Work out the finished part from the listing and answer in its coordinate system (mm). A direction names the side the tool comes from. Coordinates: 2 decimals unless noted, no trailing zeros. Loops run counter-clockwise (first coordinate to the right, second up) from the corner with the lowest first, then second, coordinate; pieces in that order, holes last. Notation, with made-up numbers: (-4.75, 74.25) -> (19.25, 74.25) arc R19 cw to (19.25, 100.25) -> close; hole circle Ø10 at (5, -10). An arc over 180 degrees is marked (long way). One line per question, with ' | ' between items.
```python
from build123d import *

# Parameters (mm, degrees)
F0_R     = 10
F0_R_2   = 5
F1_DEPTH = 10
F3_DEPTH = 15
F4_W     = 10
F4_H     = 5
F5_DEPTH = 35.001


with BuildPart() as f1:
    # F0 (on Front) → F1 (new body, symmetric)
    with BuildSketch(Plane.XZ):
        Circle(F0_R)
        Circle(F0_R_2, mode=Mode.SUBTRACT)
    extrude(amount=F1_DEPTH, both=True)

    # F2 (on face) → F3 (join)
    with BuildSketch(Plane(origin=(0, 10, 0), x_dir=(-1, 0, 0), z_dir=(0, 1, 0))):
        with BuildLine():
            ThreePointArc((0, -10), (-10, 0), (0, 10))
            Line((0, 10), (-20, 10))
            Line((-20, 10), (-25, 5))
            Line((-25, 5), (-25, -5))
            Line((-25, -5), (-20, -10))
            Line((-20, -10), (0, -10))
        make_face()
    extrude(amount=-F3_DEPTH)

    # F4 (on face) → F5 (cut, through all)
    with BuildSketch(Plane.YZ.offset(25)):
        with Locations((-5, 0)):
            Rectangle(F4_W, F4_H)
    extrude(amount=-F5_DEPTH, mode=Mode.SUBTRACT)


solid = f1.part
```
1) Find section A-A (z = 0). Write down the section's boundary in (x, y), plus the area to 3 significant figures.
Check values:
outline: (-10, 0) -> (-5, 0) -> (-5, 10) -> (-10, 10) -> close; (5, 0) -> (25, 0) -> (25, 10) -> (5, 10) -> close | area: 250 mm^2
2) Find section D-D (x = 10.5). Write down the section's boundary in (y, z).
Check values:
outline: (-5, -10) -> (10, -10) -> (10, 10) -> (-5, 10) -> (-5, 2.5) -> (0, 2.5) -> (0, -2.5) -> (-5, -2.5) -> close
3) For faces 1 (the face through (10, 3, -10)), 2 (the face through (13, -3, -2.5)), determine the directions among +Z, -Z, +X, -X, +Y, -Y from which every point of the face is accessible in a straight line to the end or side of a thin tool.
Check values:
face 1: -Z, +X, -X, +Y, -Y | face 2: +X, -X, -Y
4) The mould has two halves that part along Z. Classify faces 3 (the face through (-7, -5, 2.5)), 4 (the face through (10, 3, 10)), 5 (the face through (-10, 2, 0)): released by +Z, released by -Z, zero draft, split by the parting line, or undercut.
Check values:
face 3: undercut | face 4: released by +Z | face 5: split by the parting line
5) Find section B-B (y = 8.25). Write down the section's boundary in (x, z).
Check values:
outline: (0, -10) -> (20, -10) -> (25, -5) -> (25, 5) -> (20, 10) -> (0, 10) arc R10 ccw to start; hole circle Ø10 at (0, 0)
6) Find section C-C (y = -6.25). Write down the section's boundary in (x, z).
Check values:
outline: (-9.68, -2.5) arc R10 ccw to (9.68, -2.5) -> (4.33, -2.5) arc R5 cw to (-4.33, -2.5) -> close; (-9.68, 2.5) -> (-4.33, 2.5) arc R5 cw to (4.33, 2.5) -> (9.68, 2.5) arc R10 ccw to start
7) Find the intervals of material crossed by line 1 along X through (y, z) = (3.25, 0); line 2 along X through (y, z) = (0.25, 2.5); line 3 along Z through (x, y) = (12.5, -1), in increasing order.
Check values:
line 1: x = -10 to -5, 5 to 25 | line 2: x = -9.68 to -4.33, 4.33 to 25 | line 3: z = -10 to -2.5, 2.5 to 10
8) Flat-ended cylindrical pins translate along their axes: pin 1 (1 mm diameter, centred on x = 15.5, z = -6, fed in from -Y); pin 2 (2.5 mm diameter, centred on x = -7, z = -1, fed in from -Y); pin 3 (6 mm diameter, centred on x = -7, y = -4, fed in from +Z). Find the tip coordinate at first contact, or state that the pin passes through.
Check values:
pin 1: stops at y = -5 | pin 2: stops at y = 0 | pin 3: stops at z = 9.17
